```python
from build123d import *

# Parameters (mm, degrees)
SKETCH_1_W              = 337.35
SKETCH_1_H              = 116.87
SKETCH_1_W_2            = 324.05
SKETCH_1_H_2            = 103.07
EXTRUDE_1_DEPTH         = 8
FILLET_1_R              = 5
HOLE_WIZARD_3_2_3_2_1_D = 3.2
SKETCH_5_W              = 32
SKETCH_5_H              = 1.5
CUT_EXTRUDE_1_DEPTH     = 355.911853
EXTRUDE_2_REACH         = 356.912
SKETCH_6_W              = 3
SKETCH_6_H              = 8
SKETCH_7_W              = 257.05
SKETCH_7_H              = 8
EXTRUDE_3_DEPTH         = 4
SKETCH_8_W              = 257.05
SKETCH_8_H              = 4
EXTRUDE_4_DEPTH         = 3
SKETCH_11_W             = 99.07
SKETCH_11_H             = 11
EXTRUDE_5_DEPTH         = 2
SKETCH_13_W             = 42
SKETCH_13_H             = 4.5
CUT_EXTRUDE_2_DEPTH     = 354.692894189
SKETCH_14_W             = 121.5
SKETCH_14_H             = 1.5
CUT_EXTRUDE_3_DEPTH     = 355.911853
SKETCH_16_W             = 32
SKETCH_16_H             = 6.5
EXTRUDE_7_DEPTH         = 4
SKETCH_17_W             = 103.07
SKETCH_17_H             = 3
CUT_EXTRUDE_4_DEPTH     = 0.1
EXTRUDE_8_DEPTH         = 2
SKETCH_19_W             = 70.55
SKETCH_19_H             = 2
SKETCH_19_W_2           = 95
EXTRUDE_9_DEPTH         = 3
SKETCH_20_R             = 3.5
CUT_EXTRUDE_5_DEPTH     = 4
SKETCH_21_R             = 3.1
CUT_EXTRUDE_6_DEPTH     = 2
EXTRUDE_10_DEPTH        = 2
EXTRUDE_10_DEPTH_BACK   = 3
SKETCH_22_W             = 6
SKETCH_22_H             = 6
SKETCH_22_R             = 1.5
SKETCH_23_W             = 10
SKETCH_23_H             = 1.5
SKETCH_23_W_2           = 15
CUT_EXTRUDE_7_DEPTH     = 6.9
SKETCH_24_W             = 103.07
SKETCH_24_H             = 3
CUT_EXTRUDE_8_DEPTH     = 358.110094229
SKETCH_25_W             = 402.768513644
SKETCH_25_H             = 192.082702388
SKETCH_25_W_2           = 190
SKETCH_25_H_2           = 48.964424343
CUT_EXTRUDE_9_DEPTH     = 358.110094229
CHAMFER_1_SIZE          = 5
SKETCH_26_W             = 121.5
SKETCH_26_H             = 8.9
EXTRUDE_11_DEPTH        = 1.5


with BuildPart() as part:
    # 草图1 → 凸台-拉伸1 (new body)
    with BuildSketch(Plane(origin=(0, 0, 0), x_dir=(1, 0, 0), z_dir=(0, 1, 0))):
        with Locations((168.675, 58.435)):
            Rectangle(SKETCH_1_W, SKETCH_1_H)
        with Locations((168.925, 58.435)):
            Rectangle(SKETCH_1_W_2, SKETCH_1_H_2, mode=Mode.SUBTRACT)
    extrude(amount=EXTRUDE_1_DEPTH)

    # 圆角1
    fillet_1_edges = [part.edges().sort_by_distance(p)[0] for p in [
        (0, 4, -116.87),
        (337.35, 4, -116.87),
        (337.35, 4, 0),
        (0, 4, 0),
    ]]
    fillet(fillet_1_edges, radius=FILLET_1_R)

    # Ø3.2 (3.2) 直径孔1 (through all)
    with Locations(Plane(origin=(0, 8, 0), x_dir=(1, 0, 0), z_dir=(0, 1, 0))):
        with Locations((3.45, 98.435), (87.17, 113.42), (247.17, 113.42), (334.15, 98.435), (334.15, 18.435), (247.17, 3.45), (87.17, 3.45), (3.45, 18.435)):
            Hole(HOLE_WIZARD_3_2_3_2_1_D / 2)

    # 草图5 → 切除-拉伸1 (cut, through all)
    with BuildSketch(Plane.XY.offset(-109.97)):
        with Locations((57.9, 0.75)):
            Rectangle(SKETCH_5_W, SKETCH_5_H)
    extrude(amount=-CUT_EXTRUDE_1_DEPTH, mode=Mode.SUBTRACT)

    # 草图6 → 凸台-拉伸2 (add, up to next)
    with BuildSketch(Plane.XY.offset(-109.97), mode=Mode.PRIVATE) as extrude_2_sk1:
        with Locations((40.4, 4)):
            Rectangle(SKETCH_6_W, SKETCH_6_H)
    extrude_2_tool1 = extrude(extrude_2_sk1.sketch, amount=EXTRUDE_2_REACH, mode=Mode.PRIVATE) - part.part
    add(extrude_2_tool1.solids().sort_by_distance((40.4, 4, -109.97))[0])

    # 草图7 → 凸台-拉伸3 (add)
    with BuildSketch(Plane.XY.offset(-109.97)):
        with Locations((202.425, 4)):
            Rectangle(SKETCH_7_W, SKETCH_7_H)
    extrude(amount=EXTRUDE_3_DEPTH)

    # 草图8 → 凸台-拉伸4 (add)
    with BuildSketch(Plane.XZ):
        with Locations((202.425, -107.97)):
            Rectangle(SKETCH_8_W, SKETCH_8_H)
    extrude(amount=EXTRUDE_4_DEPTH)

    # 草图11 → 凸台-拉伸5 (add)
    with BuildSketch(Plane.ZY.offset(-330.95)):
        with Locations((-56.435, 2.5)):
            Rectangle(SKETCH_11_W, SKETCH_11_H)
    extrude(amount=EXTRUDE_5_DEPTH)

    # 草图13 → 切除-拉伸2 (cut, through all)
    with BuildSketch(Plane.XY.offset(-105.97)):
        with Locations((307.95, -0.75)):
            Rectangle(SKETCH_13_W, SKETCH_13_H)
    extrude(amount=-CUT_EXTRUDE_2_DEPTH, mode=Mode.SUBTRACT)

    # 草图14 → 切除-拉伸3 (cut, through all)
    with BuildSketch(Plane(origin=(0, 0, -6.9), x_dir=(-1, 0, 0), z_dir=(0, 0, -1))):
        with Locations((-173.2, 0.75)):
            Rectangle(SKETCH_14_W, SKETCH_14_H)
    extrude(amount=-CUT_EXTRUDE_3_DEPTH, mode=Mode.SUBTRACT)

    # 草图16 → 凸台-拉伸7 (add)
    with BuildSketch(Plane.XY.offset(-109.97)):
        with Locations((57.9, 4.75)):
            Rectangle(SKETCH_16_W, SKETCH_16_H)
    extrude(amount=EXTRUDE_7_DEPTH)

    # 草图17 → 切除-拉伸4 (cut)
    with BuildSketch(Plane(origin=(330.95, 0, 0), x_dir=(0, 0, -1), z_dir=(1, 0, 0))):
        with Locations((58.435, -1.5)):
            Rectangle(SKETCH_17_W, SKETCH_17_H)
    extrude(amount=-CUT_EXTRUDE_4_DEPTH, mode=Mode.SUBTRACT)

    # 草图18 → 凸台-拉伸8 (add)
    with BuildSketch(Plane(origin=(0, 0, -6.9), x_dir=(-1, 0, 0), z_dir=(0, 0, -1))):
        Polygon((-233.95, 0), (-233.95, 1.5), (-112.45, 1.5), (-112.45, 0), (-41.9, 0), (-41.9, 8), (-328.95, 8), (-328.95, 0), align=None)
    extrude(amount=EXTRUDE_8_DEPTH)

    # 草图19 → 凸台-拉伸9 (add)
    with BuildSketch(Plane.XZ):
        with Locations((77.175, -7.9)):
            Rectangle(SKETCH_19_W, SKETCH_19_H)
        with Locations((281.45, -7.9)):
            Rectangle(SKETCH_19_W_2, SKETCH_19_H)
    extrude(amount=EXTRUDE_9_DEPTH)

    # 草图20 → 切除-拉伸5 (cut)
    with BuildSketch(Plane.XZ.offset(3)):
        with Locations((92.088456012, -9.54)):
            Circle(SKETCH_20_R)
        with Locations((262.268456012, -9.54)):
            Circle(SKETCH_20_R)
        with Locations((328.308456012, -13.35)):
            Circle(SKETCH_20_R)
        with Locations((328.308456012, -74.31)):
            Circle(SKETCH_20_R)
        with Locations((137.808456012, -107.33)):
            Circle(SKETCH_20_R)
        with Locations((22.238456012, -9.54)):
            Circle(SKETCH_20_R)
        with Locations((9.538456012, -23.51)):
            Circle(SKETCH_20_R)
        with Locations((9.538456012, -103.52)):
            Circle(SKETCH_20_R)
    extrude(amount=-CUT_EXTRUDE_5_DEPTH, mode=Mode.SUBTRACT)

    # 草图21 → 切除-拉伸6 (cut)
    with BuildSketch(Plane(origin=(0, 8, 0), x_dir=(1, 0, 0), z_dir=(0, 1, 0))):
        with Locations(Location((87.17, 113.42, 0), (0, 0, 270))):
            Circle(SKETCH_21_R)
        with Locations(Location((247.17, 113.42, 0), (0, 0, 270))):
            Circle(SKETCH_21_R)
        with Locations(Location((334.15, 98.435, 0), (0, 0, 270))):
            Circle(SKETCH_21_R)
        with Locations(Location((334.15, 18.435, 0), (0, 0, 270))):
            Circle(SKETCH_21_R)
        with Locations(Location((247.17, 3.45, 0), (0, 0, 270))):
            Circle(SKETCH_21_R)
        with Locations(Location((87.17, 3.45, 0), (0, 0, 270))):
            Circle(SKETCH_21_R)
        with Locations(Location((3.45, 18.435, 0), (0, 0, 270))):
            Circle(SKETCH_21_R)
        with Locations(Location((3.45, 98.435, 0), (0, 0, 270))):
            Circle(SKETCH_21_R)
    extrude(amount=-CUT_EXTRUDE_6_DEPTH, mode=Mode.SUBTRACT)

    # 草图22 → 凸台-拉伸10 (add, two sides: drawn at the far end of the back side and taken through both)
    # profile 1 of 4: a face of its own
    with BuildSketch(Plane(origin=(0, 4, 0), x_dir=(1, 0, 0), z_dir=(0, 1, 0)).offset(-EXTRUDE_10_DEPTH_BACK)):
        with Locations((9.9, 106.97)):
            Rectangle(SKETCH_22_W, SKETCH_22_H)
        with Locations(Location((9.9, 106.97, 0), (0, 0, 90))):
            Circle(SKETCH_22_R, mode=Mode.SUBTRACT)
    # profile 2 of 4: a face of its own
    with BuildSketch(Plane(origin=(0, 4, 0), x_dir=(1, 0, 0), z_dir=(0, 1, 0)).offset(-EXTRUDE_10_DEPTH_BACK)):
        with Locations((35.9, 106.97)):
            Rectangle(SKETCH_22_W, SKETCH_22_H)
        with Locations(Location((35.9, 106.97, 0), (0, 0, 90))):
            Circle(SKETCH_22_R, mode=Mode.SUBTRACT)
    # profile 3 of 4: a face of its own
    with BuildSketch(Plane(origin=(0, 4, 0), x_dir=(1, 0, 0), z_dir=(0, 1, 0)).offset(-EXTRUDE_10_DEPTH_BACK)):
        with Locations((9.9, 9.9)):
            Rectangle(SKETCH_22_W, SKETCH_22_H)
        with Locations(Location((9.9, 9.9, 0), (0, 0, 90))):
            Circle(SKETCH_22_R, mode=Mode.SUBTRACT)
    # profile 4 of 4: a face of its own
    with BuildSketch(Plane(origin=(0, 4, 0), x_dir=(1, 0, 0), z_dir=(0, 1, 0)).offset(-EXTRUDE_10_DEPTH_BACK)):
        with Locations((35.9, 9.9)):
            Rectangle(SKETCH_22_W, SKETCH_22_H)
        with Locations(Location((35.9, 9.9, 0), (0, 0, 90))):
            Circle(SKETCH_22_R, mode=Mode.SUBTRACT)
    extrude(amount=EXTRUDE_10_DEPTH + EXTRUDE_10_DEPTH_BACK)

    # 草图23 → 切除-拉伸7 (cut)
    with BuildSketch(Plane.ZY):
        with Locations((-63.435, 0.75)):
            Rectangle(SKETCH_23_W, SKETCH_23_H)
        with Locations((-50.935, 0.75)):
            Rectangle(SKETCH_23_W_2, SKETCH_23_H)
    extrude(amount=-CUT_EXTRUDE_7_DEPTH, mode=Mode.SUBTRACT)

    # 草图24 → 切除-拉伸8 (cut, through all)
    with BuildSketch(Plane(origin=(337.35, 0, 0), x_dir=(0, 0, -1), z_dir=(1, 0, 0))):
        with Locations((58.435, -1.5)):
            Rectangle(SKETCH_24_W, SKETCH_24_H)
    extrude(amount=-CUT_EXTRUDE_8_DEPTH, mode=Mode.SUBTRACT)

    # 草图25 → 切除-拉伸9 (cut, through all)
    with BuildSketch(Plane(origin=(0, 8, 0), x_dir=(1, 0, 0), z_dir=(0, 1, 0))):
        with Locations((167.276381716, 50.966242561)):
            Rectangle(SKETCH_25_W, SKETCH_25_H)
        with Locations((167.17, 6.206921893)):
            Rectangle(SKETCH_25_W_2, SKETCH_25_H_2, mode=Mode.SUBTRACT)
    extrude(amount=-CUT_EXTRUDE_9_DEPTH, mode=Mode.SUBTRACT)

    # 倒角1
    chamfer_1_edges = [part.edges().sort_by_distance(p)[0] for p in [
        (72.17, 8, -4.45),
        (262.17, 8, -4.45),
    ]]
    chamfer(chamfer_1_edges, length=CHAMFER_1_SIZE)

    # 草图26 → 凸台-拉伸11 (add)
    with BuildSketch(Plane.XZ.offset(-1.5)):
        with Locations((173.2, -4.45)):
            Rectangle(SKETCH_26_W, SKETCH_26_H)
    extrude(amount=EXTRUDE_11_DEPTH)


solid = part.part
```
Input: part model. Units: mm. Frame: model coordinates. A direction names the side the tool comes from. Give positions to 0.01 mm unless a question says otherwise; leave off trailing zeros. Order: outer loops, then holes, each group sorted by start corner. A loop starts at its lowest first (then second) coordinate and runs counter-clockwise, first axis right, second up. Notation, with made-up numbers: M 0.25,-13 L 11.25,-13 A21 ccw 11.25,7 Z; hole C 86.5,33 d4. An arc over 180 degrees is marked long. Return JSON: item names as keys, results as strings.
Item 1: First-contact query: P1, Ø2.5, axis at x = 92, z = -7.5, coming from the -Y side; P2, Ø5, axis at x = 175, z = -8, coming from the -Y side; P3, Ø3, axis at x = 246.5, z = -2.5, coming from the +Y side. Flat tips, straight axial feed; report the tip coordinate or a pass-through.
Solutions:
{"P1": "y = 1", "P2": "y = 0", "P3": "y = 6"}
Item 2: Cut plane B-B (x = 247.17). Return loops of the section in (y, z).
Solutions:
{"outline": "M 0,-8.9 L 8,-8.9 L 8,-6.55 L 6,-6.55 L 6,-5.05 L 0,-5.05 Z; M 0,-1.85 L 6,-1.85 L 6,-0.35 L 8,-0.35 L 8,0 L 0,0 Z"}
Item 3: Access query for faces 4 (the cylindrical face through (250.244, 7.014, -3.854)), 5 (the cylindrical face through (260.02, 0.49, -6.86)), 6 (the flat face through (92, 1, -8)). Directions: +Z, -Z, +X, -X, +Y, -Y. A direction counts if a zero-diameter tool reaches every point of the face in a straight line with its end or side. Return the directions, or none.
Solutions:
{"face 4": "+Y", "face 5": "-Z, +X, -Y", "face 6": "-Z, -Y"}
Item 4: Cut plane C-C (y = 4.5). Return loops of the section in (x, z).
Solutions:
{"outline": "M 73.67,-8.9 L 260.67,-8.9 L 260.67,0 L 73.67,0 Z; hole C 87.17,-3.45 d3.2; hole C 247.17,-3.45 d3.2"}
Item 5: Ray query, probe 1 along Z at (x, y) = (87.17, 3.45); probe 2 along X at (y, z) = (0.5, -3.25); probe 3 along X at (y, z) = (7.2, -3.45). Return the intervals inside material, ascending.
Solutions:
{"probe 1": "-8.9 to -5.05, -1.85 to 0", "probe 2": "72.17 to 85.58, 88.76 to 245.58, 248.76 to 262.17", "probe 3": "76.37 to 84.07, 90.27 to 244.07, 250.27 to 257.97"}
Item 6: Pull-direction query (Z, two-part tool) for faces 1 (the flat face through (261, 1, -8)), 2 (the flat face through (166, 4, -8.9)), 3 (the flat face through (246, 6, -2)); classes: +Z half, -Z half, draft (parallel to the pull), parting line (faces both ways), or undercut.
Solutions:
{"face 1": "draft", "face 2": "-Z half", "face 3": "undercut"}
Item 7: Cut plane A-A (z = -3.45). Return loops of the section in (x, y), then the cut area to 3 significant figures.
Solutions:
{"outline": "M 72.17,0 L 85.57,0 L 85.57,6 L 84.07,6 L 84.07,8 L 77.17,8 L 72.17,3 Z; M 88.77,0 L 245.57,0 L 245.57,6 L 244.07,6 L 244.07,8 L 90.27,8 L 90.27,6 L 88.77,6 Z; M 248.77,0 L 262.17,0 L 262.17,3 L 257.17,8 L 250.27,8 L 250.27,6 L 248.77,6 Z", "area": "1,430 mm^2"}
